Geometry: final body of the model. Coordinates: model frame, mm. A direction names the side the tool comes from. Give positions to 0.01 mm unless a question says otherwise; leave off trailing zeros. Order: outer loops, then holes, each group sorted by start corner. A loop starts at its lowest first (then second) coordinate and runs counter-clockwise, first axis right, second up. Notation, with made-up numbers: (6, -31.75) -> (52, -31.75) arc R21 cw to (52, -3.75) -> close; hole circle Ø1 at (47, -15.5). An arc over 180 degrees is marked (long way). One line per question, with ' | ' between items.
from build123d import *

# Parameters (mm, degrees)
CUT_EXTRUDE1_REACH             = 11.908
SKETCH2_W                      = 0.41
SKETCH2_H                      = 1
CUT_EXTRUDE1_DIRECTION_2_REACH = 11.908


with BuildPart() as part:
    # Sketch1 → Revolve1 (revolve)
    with BuildSketch(Plane.XY, mode=Mode.PRIVATE) as revolve1_sk:
        with BuildLine():
            Line((0, 9), (1.93, 9))
            ThreePointArc((1.93, 9), (2.637106781, 8.707106781), (2.93, 8))
            Line((2.93, 8), (2.93, 7))
            Line((2.93, 7), (2, 7))
            Line((2, 7), (2, 0))
            Line((2, 0), (0, 0))
            Line((0, 0), (0, 9))
        make_face()
    revolve(revolve1_sk.sketch.rotate(Axis((0, 0, 0), (0, 1, 0)), 90), axis=Axis((0, 0, 0), (0, 1, 0)))

    # Sketch2 → Cut-Extrude1 (cut, up to next)
    with BuildSketch(Plane.XY, mode=Mode.PRIVATE) as cut_extrude1_sk1:
        with Locations((0, 8.5)):
            Rectangle(SKETCH2_W, SKETCH2_H)
    cut_extrude1_tool1 = extrude(cut_extrude1_sk1.sketch, amount=-CUT_EXTRUDE1_REACH, mode=Mode.PRIVATE) & part.part
    add(cut_extrude1_tool1.solids().sort_by_distance((0, 8.5, 0))[0], mode=Mode.SUBTRACT)

    # Sketch2 → Cut-Extrude1 direction 2 (cut, up to next)
    with BuildSketch(Plane.XY, mode=Mode.PRIVATE) as cut_extrude1_direction_2_sk1:
        with Locations((0, 8.5)):
            Rectangle(SKETCH2_W, SKETCH2_H)
    cut_extrude1_direction_2_tool1 = extrude(cut_extrude1_direction_2_sk1.sketch, amount=CUT_EXTRUDE1_DIRECTION_2_REACH, mode=Mode.PRIVATE) & part.part
    add(cut_extrude1_direction_2_tool1.solids().sort_by_distance((0, 8.5, 0))[0], mode=Mode.SUBTRACT)


solid = part.part
1) Section A-A on x = 0. Return loops of the section in (y, z), plus the area to 3 significant figures.
Check result:
outline: (0, -2) -> (7, -2) -> (7, -2.93) -> (8, -2.93) -> (8, 2.93) -> (7, 2.93) -> (7, 2) -> (0, 2) -> close | area: 33.9 mm^2
2) Section C-C on y = 8.25. Return loops of the section in (x, z) (1 decimal).
Check result:
outline: (-0.2, -2.9) -> (-0.2, 2.9) arc R2.9 ccw to start; (0.2, -2.9) arc R2.9 ccw to (0.2, 2.9) -> close
3) Pull-direction query (X, two-part tool) for faces 1 (the flat face through (0.205, 8.5, 0)), 2 (the flat face through (0, 0, 0)), 3 (the flat face through (-0.205, 8.5, 0)), 4 (the cylindrical face through (2, 3, 0)); classes: +X half, -X half, draft (parallel to the pull), parting line (faces both ways), or undercut.
Check result:
face 1: undercut | face 2: draft | face 3: undercut | face 4: parting line
4) Material intervals for probe 1 along Y at (x, z) = (0.15, -2.45); probe 2 along X at (y, z) = (7.75, -0.1); probe 3 along X at (y, z) = (6, -0.35), sorted ascending. Write a range as from..to.
Check result:
probe 1: y = 7..8 | probe 2: x = -2.93..2.93 | probe 3: x = -1.97..1.97
5) Section B-B on z = 0. Return loops of the section in (x, y) (3 decimals), plus the area to 3 significant figures.
Check result:
outline: (-2.93, 7) -> (-2, 7) -> (-2, 0) -> (2, 0) -> (2, 7) -> (2.93, 7) -> (2.93, 8) arc R1 ccw to (1.93, 9) -> (0.205, 9) -> (0.205, 8) -> (-0.205, 8) -> (-0.205, 9) -> (-1.93, 9) arc R1 ccw to (-2.93, 8) -> close | area: 38.9 mm^2
6) Contact query for flat-ended pins moving along their axis: pin 1 Ø1.5 at (x, y) = (-1.5, 7) entering from +Z; pin 2 Ø0.5 at (y, z) = (8.5, -0.5) entering from +X; pin 3 Ø3 at (y, z) = (6, -2) entering from +X. Output: stop coordinate, or through.
Check result:
pin 1: stops at z = 2.83 | pin 2: stops at x = 2.86 | pin 3: stops at x = 2.79
7) Set-up query: faces 5 (the flat face through (-1, 9, 0)), 6 (the flat face through (2, 7, -1)). Return all of +Z, -Z, +X, -X, +Y, -Y with unobstructed straight access to the full face (end or side cutting, diameter ignored); none if empty.
Check result:
face 5: +Z, -Z, +X, -X, +Y | face 6: -Y
8) Section D-D on y = 1.25. Return loops of the section in (x, z).
Check result:
outline: circle Ø4 at (0, 0)
